Check sheet for the modelled part. Datum: model origin and axes. Units: mm. Give positions to 0.01 mm unless a question says otherwise; leave off trailing zeros. Loops run counter-clockwise (first coordinate to the right, second up) from the corner with the lowest first, then second, coordinate; pieces in that order, holes last. Notation, with made-up numbers: (20, 27.25) -> (41, 27.25) arc R13 ccw to (41, 52.25) -> close; hole circle Ø2 at (72.5, 48.25). An arc over 180 degrees is marked (long way). Write each question's results on one line, items separated by ' | '. Start each with the question number.
Item 1: Cross-section at A-A on x = 0. Enter the section's corners in (y, z) (3 decimals), then the cut area to 4 significant figures.
Item 2: Cross-section at C-C on x = 1.45. Enter the section's corners in (y, z).
Item 3: Cross-section at B-B on z = 0.6. Enter the section's corners in (x, y) (3 decimals), then the cut area to 3 significant figures.
Item 4: Scan lines: line 1 along Y through (x, z) = (0, 0.55) (3 decimals); line 2 along Y through (x, z) = (-0.85, 0.6); line 3 along Y through (x, z) = (-1.5, 0.65). Record each from-to range of solid material in increasing order.
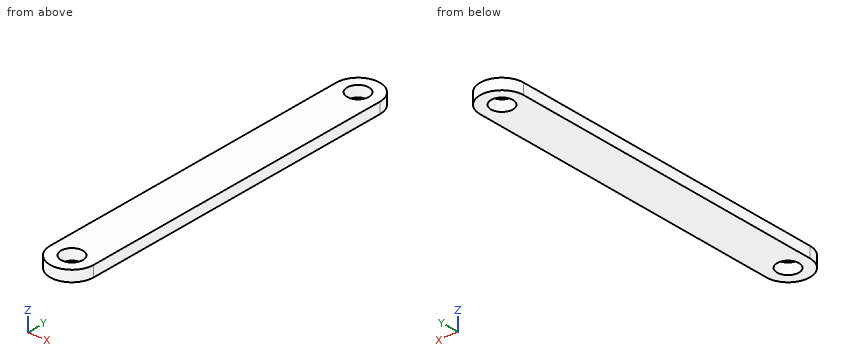
Autodesk Inventor part; units mm, degrees
ref_plane "YZ Plane" through (0, 0, 0) normal (1, 0, 0) x (0, 1, 0)
ref_plane "XZ Plane" through (0, 0, 0) normal (0, 1, 0) x (-1, 0, 0)
ref_plane "XY Plane" through (0, 0, 0) normal (0, 0, 1) x (1, 0, 0)
sketch "草圖1" plane through (0, 0, 0) normal (0, 0, 1) x (1, 0, 0)
  line L0 (0, -14.975) -> (0, 14.975) construction
  line L1 (2, -14.975) -> (2, 14.975)
  line L2 (-2, 14.975) -> (-2, -14.975)
  arc A0 (-2, -14.975) -> (2, -14.975) centre (0, -14.975) ccw
  arc A1 (2, 14.975) -> (-2, 14.975) centre (0, 14.975) ccw
  point P0 (0, 0)
  dimension "d0" = 29.95
  dimension "d1" = 4
extrude "擠出1" add sketch "草圖1" along normal blind 1
sketch "草圖2" plane through (0, 0, 1) normal (0, 0, 1) x (1, 0, 0)
  arc A0 (2, 14.975) -> (-2, 14.975) centre (0, 14.975) ccw
  circle A1 centre (0, 14.975) radius 0.75
  arc A2 (-2, -14.975) -> (2, -14.975) centre (0, -14.975) ccw
  circle A3 centre (0, -14.975) radius 0.75
  point P0 (0, 0)
  dimension "d6" = 1.5
  dimension "d7" = 1.5
extrude "擠出2" add sketch "草圖2" along normal blind 1
sketch "草圖3" plane through (0, 0, 1) normal (0, 0, 1) x (1, 0, 0)
  circle A0 centre (0, 14.975) radius 0.75
  circle A1 centre (0, 14.975) radius 1
  circle A2 centre (0, -14.975) radius 0.75
  circle A3 centre (0, -14.975) radius 1
  point P0 (0, 0)
  dimension "d10" = 2
  dimension "d11" = 2
extrude "擠出3" cut sketch "草圖3" along normal mid plane 10 contours A0 | A1 | A2 | A3
properties part number "連桿1"
Answer sheet:
1) outline: (-16.975, 0) -> (-15.975, 0) -> (-15.975, 1) -> (-16.975, 1) -> close; (-13.975, 0) -> (13.975, 0) -> (13.975, 1) -> (-13.975, 1) -> close; (15.975, 0) -> (16.975, 0) -> (16.975, 1) -> (15.975, 1) -> close | area: 29.95 mm²
2) outline: (-16.35, 0) -> (16.35, 0) -> (16.35, 1) -> (-16.35, 1) -> close
3) outline: (-2, -14.975) arc R2 ccw to (2, -14.975) -> (2, 14.975) arc R2 ccw to (-2, 14.975) -> close; hole circle Ø2 at (0, -14.975); hole circle Ø2 at (0, 14.975) | area: 126 mm²
4) line 1: y = -16.975 to -15.975, -13.975 to 13.975, 15.975 to 16.975 | line 2: y = -16.79 to -15.5, -14.45 to 14.45, 15.5 to 16.79 | line 3: y = -16.3 to 16.3
